Geometry check sheet. Reference: drawing and pictorial views, mm from the part's lowest x, y, z. Round coordinates to 2 decimals unless told otherwise and drop trailing zeros. Order: outer loops, then holes, each group sorted by start corner. A loop starts at its lowest first (then second) coordinate and runs counter-clockwise, first axis right, second up.
(1) Thickness scan on L1, parallel to Y at x = 60, z = 7.5; L2, parallel to X at y = 4, z = 6; L3, parallel to Y at x = 57.5, z = 10.5. Record the ranges inside material, lowest first.
(2) Cross-section at B-B on z = 6. Enter the section's corners in (x, y).
(3) Gauge pin test, flat ends, axial feed: P1, Ø6, axis at y = 36.5, z = 2.5, coming from the +X side; P2, Ø1.5, axis at x = 99, z = 5, coming from the -Y side. Record the tip position at first contact, or that the pin passes through.
(4) Cross-section at A-A on x = 20. Enter the section's corners in (y, z).
(5) Cross-section at C-C on x = 60. Enter the section's corners in (y, z).
(6) Cross-section at D-D on y = 110. Enter the section's corners in (x, z), and give its area (3 significant figures).
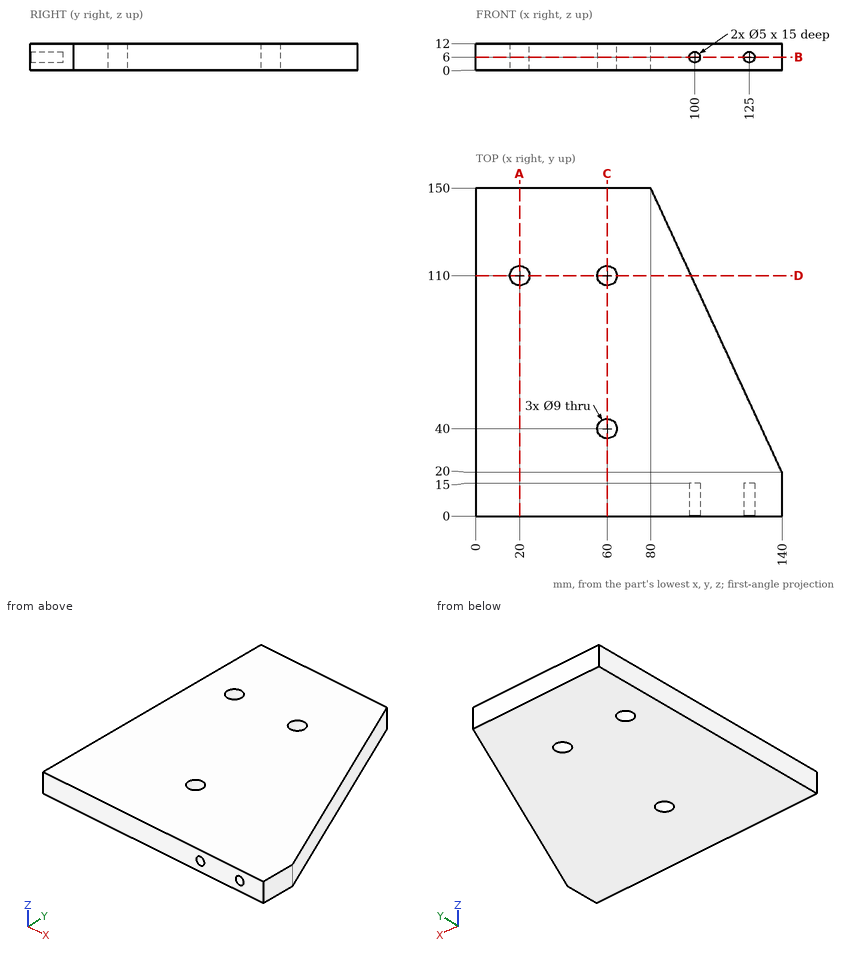
Found:
1. L1: y = 0 to 35.5, 44.5 to 105.5, 114.5 to 150
1. L2: x = 0 to 97.5, 102.5 to 122.5, 127.5 to 140
1. L3: y = 0 to 36.26, 43.74 to 106.26, 113.74 to 150
2. outline: (0, 0) - (97.5, 0) - (97.5, 15) - (102.5, 15) - (102.5, 0) - (122.5, 0) - (122.5, 15) - (127.5, 15) - (127.5, 0) - (140, 0) - (140, 20) - (80, 150) - (0, 150) - close; hole circle Ø9 at (20, 110); hole circle Ø9 at (60, 40); hole circle Ø9 at (60, 110)
3. P1: stops at x = 133.77
3. P2: stops at y = 15
4. outline: (0, 0) - (105.5, 0) - (105.5, 12) - (0, 12) - close; (114.5, 0) - (150, 0) - (150, 12) - (114.5, 12) - close
5. outline: (0, 0) - (35.5, 0) - (35.5, 12) - (0, 12) - close; (44.5, 0) - (105.5, 0) - (105.5, 12) - (44.5, 12) - close; (114.5, 0) - (150, 0) - (150, 12) - (114.5, 12) - close
6. outline: (0, 0) - (15.5, 0) - (15.5, 12) - (0, 12) - close; (24.5, 0) - (55.5, 0) - (55.5, 12) - (24.5, 12) - close; (64.5, 0) - (98.46, 0) - (98.46, 12) - (64.5, 12) - close
6. area: 966 mm2
